from build123d import *

# Parameters (mm, degrees)
SKETCH1_R              = 44.45
SKETCH1_R_2            = 38.6334
BASE_DEPTH             = 203.2
SKETCH2_W              = 31.75
SKETCH2_H              = 38.1
SANDING_CUT_DEPTH      = 45.45
SANDING_CUT_DEPTH_BACK = 45.45
SKETCH3_W              = 38.1
SKETCH3_H              = 12.7
SERVO_CUT_DEPTH        = 45.45
SERVO_CUT_DEPTH_BACK   = 45.45


with BuildPart() as part:
    # Sketch1 → base (new body)
    with BuildSketch(Plane.XY):
        Circle(SKETCH1_R)
        Circle(SKETCH1_R_2, mode=Mode.SUBTRACT)
    extrude(amount=BASE_DEPTH)

    # Sketch2 → sanding cut (cut, two sides)
    with BuildSketch(Plane(origin=(0, 0, 0), x_dir=(0, 0, -1), z_dir=(1, 0, 0))) as sanding_cut_sk:
        with Locations((-133.35, 25.4)):
            Rectangle(SKETCH2_W, SKETCH2_H)
    extrude(amount=SANDING_CUT_DEPTH, mode=Mode.SUBTRACT)
    extrude(sanding_cut_sk.sketch, amount=-SANDING_CUT_DEPTH_BACK, mode=Mode.SUBTRACT)

    # Sketch3 → servo cut (cut, two sides)
    with BuildSketch(Plane(origin=(0, 0, 0), x_dir=(0, 0, -1), z_dir=(1, 0, 0))) as servo_cut_sk:
        with Locations((-117.475, -38.1)):
            Rectangle(SKETCH3_W, SKETCH3_H)
    extrude(amount=SERVO_CUT_DEPTH, mode=Mode.SUBTRACT)
    extrude(servo_cut_sk.sketch, amount=-SERVO_CUT_DEPTH_BACK, mode=Mode.SUBTRACT)


solid = part.part
Geometry check sheet. Reference: the model listing, model coordinates, mm. A direction names the side the tool comes from. Give positions to 0.01 mm unless a question says otherwise; leave off trailing zeros. Loops run counter-clockwise (first coordinate to the right, second up) from the corner with the lowest first, then second, coordinate; pieces in that order, holes last. Notation, with made-up numbers: (3.25, 20) -> (52.25, 20) arc R34 cw to (52.25, 54) -> close; hole circle Ø6 at (-18, 74.5). An arc over 180 degrees is marked (long way). Answer in a Markdown table with one row per item. Add a question column.
1) Cross-section at C-C on y = 0. Record the boundary of the cut face in (x, z).
2) Draft check along Z on faces 4 (the face through (-13.4, 36.4, 0)), 5 (the face through (0, -40, 136.525)), 6 (the face through (-13.4, 36.4, 203.2)). Enter one of: pulls with the +Z half, pulls with the -Z half, needs draft (parallel to the pull), parting line crosses it, or undercut.
3) Gauge pin test, flat ends, axial feed: P1, Ø5, axis at x = -9, z = 72.5, coming from the -Y side; P2, Ø4, axis at x = 17.5, z = 157, coming from the +Y side; P3, Ø10, axis at y = -16, z = 29.5, coming from the +X side. Record the tip position at first contact, or that the pin passes through.
4) Set-up check for faces 1 (the face through (0, 39, 117.475)), 2 (the face through (26, -31.75, 118)), 3 (the face through (-30.658, -23.508, 100.178)): record each of +Z, -Z, +X, -X, +Y, -Y from which the full face is reachable in a straight line by a thin tool's end or side.
5) Cross-section at D-D on y = 29. Record the boundary of the cut face in (x, z) (3 decimals), and give its area (3 significant figures).
6) Cross-section at A-A on z = 124.5. Record the boundary of the cut face in (x, y).
7) Cross-section at B-B on x = 0. Record the boundary of the cut face in (y, z) (3 decimals), and give its area (3 significant figures).
8) Material ranges on probe 1 along Y at (x, z) = (0, 86); probe 2 along Y at (x, z) = (-6.5, 45.5); probe 3 along X at (y, z) = (-22, 24.5), recorded low to high. Write a range as from..to.
Outcome:
| question | item | result |
|---|---|---|
| 1 | outline | (-44.45, 0) -> (-38.63, 0) -> (-38.63, 203.2) -> (-44.45, 203.2) -> close; (38.63, 0) -> (44.45, 0) -> (44.45, 203.2) -> (38.63, 203.2) -> close |
| 2 | face 4 | pulls with the -Z half |
| 2 | face 5 | undercut |
| 2 | face 6 | pulls with the +Z half |
| 3 | P1 | stops at y = -43.97 |
| 3 | P2 | stops at y = 41.66 |
| 3 | P3 | stops at x = 43.07 |
| 4 | face 1 | +X, -X, +Y |
| 4 | face 2 | +X, -X, -Y |
| 4 | face 3 | +Z, -Z |
| 5 | outline | (-33.687, 0) -> (-25.525, 0) -> (-25.525, 117.475) -> (-33.687, 117.475) -> close; (-33.687, 149.225) -> (-25.525, 149.225) -> (-25.525, 203.2) -> (-33.687, 203.2) -> close; (25.525, 0) -> (33.687, 0) -> (33.687, 117.475) -> (25.525, 117.475) -> close; (25.525, 149.225) -> (33.687, 149.225) -> (33.687, 203.2) -> (25.525, 203.2) -> close |
| 5 | area | 2,800 mm^2 |
| 6 | outline | (-43.99, 6.35) arc R44.45 ccw to (-31.11, -31.75) -> (-22.01, -31.75) arc R38.63 cw to (-38.11, 6.35) -> close; (22.01, -31.75) -> (31.11, -31.75) arc R44.45 ccw to (43.99, 6.35) -> (38.11, 6.35) arc R38.63 cw to start |
| 7 | outline | (-44.45, 0) -> (-38.633, 0) -> (-38.633, 98.425) -> (-44.45, 98.425) -> close; (-44.45, 136.525) -> (-38.633, 136.525) -> (-38.633, 203.2) -> (-44.45, 203.2) -> close; (38.633, 0) -> (44.45, 0) -> (44.45, 117.475) -> (38.633, 117.475) -> close; (38.633, 149.225) -> (44.45, 149.225) -> (44.45, 203.2) -> (38.633, 203.2) -> close |
| 7 | area | 1,960 mm^2 |
| 8 | probe 1 | y = -44.45..-38.63, 38.63..44.45 |
| 8 | probe 2 | y = -43.97..-38.08, 38.08..43.97 |
| 8 | probe 3 | x = -38.62..-31.76, 31.76..38.62 |
